The listing builds one solid part. Answer for the finished solid, in the listing's coordinates (mm). Round coordinates to 2 decimals unless told otherwise and drop trailing zeros. Use a Markdown table: item, result. Add a question column.
1) Each of these flat-tipped pins is pushed along its axis until it touches: P1, Ø1.5, axis at x = 5.5, y = 9, coming from the +Z side; P2, Ø1.5, axis at x = 13, z = -2.5, coming from the +Y side; P3, Ø1, axis at x = 11, y = 9, coming from the +Z side; P4, Ø3.5, axis at y = 5, z = -5, coming from the -X side. Where does it stop, or does it pass through?
2) Find the intervals of material crossed by probe 1 along Z at (x, y) = (5, 5); probe 2 along Z at (x, y) = (6.75, 6.75); probe 3 along Y at (x, z) = (1.5, -5), in increasing order. Write a range as from..to.
3) Determine the mould class of faces 1 (the flat face through (8, 4, 0)), 2 (the flat face through (0, 4, -3)), 3 (the cylindrical face through (4.1, 6.2, -6.6)) for opening direction Z: +Z half, -Z half, draft (parallel to the pull), parting line (faces both ways), or undercut.
Autodesk Inventor part; units mm, degrees
ref_plane "YZ Plane" through (0, 0, 0) normal (1, 0, 0) x (0, 1, 0)
ref_plane "XZ Plane" through (0, 0, 0) normal (0, 1, 0) x (-1, 0, 0)
ref_plane "XY Plane" through (0, 0, 0) normal (0, 0, 1) x (1, 0, 0)
sketch "Sketch1" plane through (0, 0, 0) normal (0, 1, 0) x (-1, 0, 0)
  arc A0 (-1.1282, -10.942) -> (0, -11) centre (0, 0) ccw
  line L0 (0, 0) -> (0, -11)
  line L1 (0, 0) -> (-11, 0)
  line L2 (0, 0) -> (-20, 0)
  arc A1 (-20, 0) -> (0, -11) centre (0.7193, 13.9896) ccw
  dimension "d4" = 22
  dimension "d15" = 20
  dimension "d16" = 25
revolve "Revolution1" add sketch "Sketch1" angle 90 about axis through (0, 0, 0) along (1, 0, 0) contours A1 L2 L1 L0
sketch "Sketch2" plane through (0, 0, -11) normal (-1, 0, 0) x (0, 0, 1)
  line L0 (11, 0) -> (3.2218, 7.7782)
  arc A0 (11, 11) -> (0, 0) centre (11, 0) ccw
  line L1 (11, 11) -> (11, 0)
  point P0 (6, 5)
  dimension "d6" = 45
  dimension "d7" = 5
hole "Hole1" at (0, 5, -5) direction (1, 0, 0) diameter 4 depth 8 tip angle 118
properties part number "corner_insert"
Entries:
| question | item | result |
|---|---|---|
| 1 | P1 | stops at z = 0 |
| 1 | P2 | stops at y = 7.01 |
| 1 | P3 | passes through |
| 1 | P4 | stops at x = 8.15 |
| 2 | probe 1 | z = -9.06..-7, -3..0 |
| 2 | probe 2 | z = -7.2..-5.97, -4.03..0 |
| 2 | probe 3 | y = 0..3, 7..9.7 |
| 3 | face 1 | +Z half |
| 3 | face 2 | draft |
| 3 | face 3 | undercut |
